Source: three-view drawing plus pictorial views. Frame: mm from the lowest corner of the part. A direction names the side the tool comes from. Give positions to 0.01 mm unless a question says otherwise; leave off trailing zeros. Loops run counter-clockwise (first coordinate to the right, second up) from the corner with the lowest first, then second, coordinate; pieces in that order, holes last. Notation, with made-up numbers: (8.5, 77) - (60.5, 77) arc R11 cw to (60.5, 82) - close; hole circle Ø9 at (63, 69). An arc over 180 degrees is marked (long way). Answer in a Markdown table with one row per item.
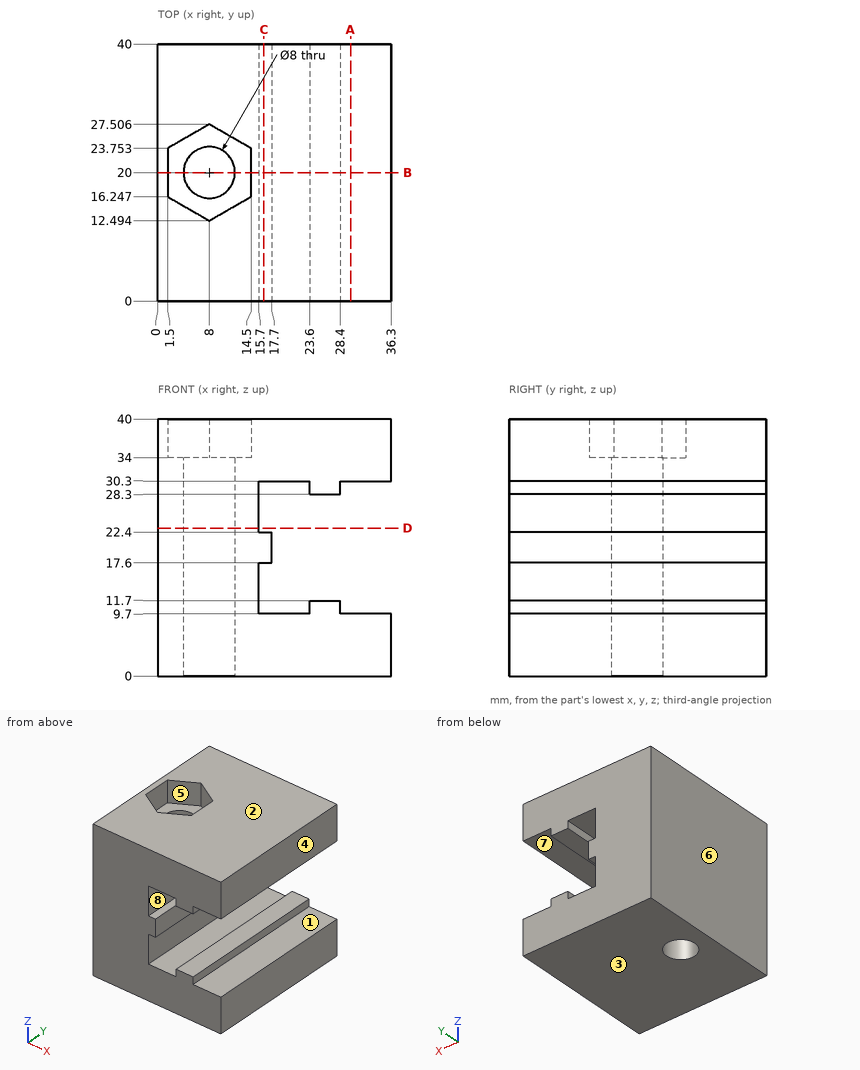
Q1. First-contact query: pin 1 (1.6 mm diameter, centred on y = 10.5, z = 29, fed in from +X); pin 2 (2.5 mm diameter, centred on y = 16.5, z = 13.5, fed in from +X); pin 3 (1.4 mm diameter, centred on y = 25, z = 19.5, fed in from +X). Flat tips, straight axial feed; report the tip coordinate or a pass-through.
Check values:
| item | result |
|---|---|
| pin 1 | x = 28.4 |
| pin 2 | x = 15.7 |
| pin 3 | x = 17.7 |
Q2. Cut plane C-C (x = 16.5). Output: boundary loops of the cut face in (y, z), and give its area (3 significant figures).
Check values:
| item | result |
|---|---|
| outline | (0, 0) - (40, 0) - (40, 9.7) - (0, 9.7) - close; (0, 17.6) - (40, 17.6) - (40, 22.4) - (0, 22.4) - close; (0, 30.3) - (40, 30.3) - (40, 40) - (0, 40) - close |
| area | 968 mm² |
Q3. Draft query along Z for the marked faces 1, 2, 3 and 4. Return one class per face: pulls with the +Z half, pulls with the -Z half, needs draft (parallel to the pull), parting line crosses it, or undercut.
Check values:
| item | result |
|---|---|
| face 1 | undercut |
| face 2 | pulls with the +Z half |
| face 3 | pulls with the -Z half |
| face 4 | needs draft |
Q4. Cut plane D-D (z = 23). Output: boundary loops of the cut face in (x, y).
Check values:
| item | result |
|---|---|
| outline | (0, 0) - (15.7, 0) - (15.7, 40) - (0, 40) - close; hole circle Ø8 at (8, 20) |
Q5. Reachability of the marked faces 5, 6, 7 and 8 from +Z, -Z, +X, -X, +Y, -Y: full face, straight path, thin tool, end or side. Return the list, or none.
Check values:
| item | result |
|---|---|
| face 5 | +Z |
| face 6 | +Z, -Z, -X, +Y, -Y |
| face 7 | +X, +Y, -Y |
| face 8 | +Y, -Y |
Q6. Cut plane B-B (y = 20). Output: boundary loops of the cut face in (x, z).
Check values:
| item | result |
|---|---|
| outline | (0, 0) - (4, 0) - (4, 34) - (1.5, 34) - (1.5, 40) - (0, 40) - close; (12, 0) - (36.3, 0) - (36.3, 9.7) - (28.4, 9.7) - (28.4, 11.7) - (23.6, 11.7) - (23.6, 9.7) - (15.7, 9.7) - (15.7, 17.6) - (17.7, 17.6) - (17.7, 22.4) - (15.7, 22.4) - (15.7, 30.3) - (23.6, 30.3) - (23.6, 28.3) - (28.4, 28.3) - (28.4, 30.3) - (36.3, 30.3) - (36.3, 40) - (14.5, 40) - (14.5, 34) - (12, 34) - close |
Q7. Cut plane A-A (x = 30). Output: boundary loops of the cut face in (y, z).
Check values:
| item | result |
|---|---|
| outline | (0, 0) - (40, 0) - (40, 9.7) - (0, 9.7) - close; (0, 30.3) - (40, 30.3) - (40, 40) - (0, 40) - close |
Q8. Material intervals for line 1 along Y through (x, z) = (8, 23.5); line 2 along X through (y, z) = (33.5, 28.5); line 3 along X through (y, z) = (23, 38), sorted ascending.
Check values:
| item | result |
|---|---|
| line 1 | 0 to 16, 24 to 40 |
| line 2 | 0 to 15.7, 23.6 to 28.4 |
| line 3 | 0 to 1.5, 14.5 to 36.3 |
